```python
from build123d import *

# Parameters (mm, degrees)
IZIM1_W                     = 72
IZIM1_H                     = 72
Y_KSEKLIK_EKSTR_ZYON1_DEPTH = 340


with BuildPart() as part:
    # Çizim1 → Yükseklik-Ekstrüzyon1 (new body)
    with BuildSketch(Plane.XY):
        with BuildLine():
            Line((-36, 40), (36, 40))
            ThreePointArc((36, 40), (38.828427125, 38.828427125), (40, 36))
            Line((40, 36), (40, -36))
            ThreePointArc((40, -36), (38.828427125, -38.828427125), (36, -40))
            Line((36, -40), (-36, -40))
            ThreePointArc((-36, -40), (-38.828427125, -38.828427125), (-40, -36))
            Line((-40, -36), (-40, 36))
            ThreePointArc((-40, 36), (-38.828427125, 38.828427125), (-36, 40))
        make_face()
        Rectangle(IZIM1_W, IZIM1_H, mode=Mode.SUBTRACT)
    extrude(amount=Y_KSEKLIK_EKSTR_ZYON1_DEPTH)


solid = part.part
```
Geometry: final body of the model. Coordinates: model frame, mm. A direction names the side the tool comes from. Round coordinates to 2 decimals unless told otherwise and drop trailing zeros. Order: outer loops, then holes, each group sorted by start corner. A loop starts at its lowest first (then second) coordinate and runs counter-clockwise, first axis right, second up. Notation, with made-up numbers: (-7.75, 2) - (29.25, 2) arc R23 ccw to (29.25, 21) - close; hole circle Ø5 at (34.25, 77). An arc over 180 degrees is marked (long way). Write item = value, one per line. Start each with the question number.
Q1. Access query for faces 4 (the flat face through (40, 1, 168)), 5 (the flat face through (-1, 36, 168)). Directions: +Z, -Z, +X, -X, +Y, -Y. A direction counts if a zero-diameter tool reaches every point of the face in a straight line with its end or side. Return the directions, or none.
Q2. Ray query, line 1 (X direction, y = -7, z = 54); line 2 (Y direction, x = -37, z = 54). Return the intervals inside material, ascending. Write a range as from..to.
Q3. Cut plane A-A on x = 6.5. Return the cut outline in (y, z).
Q4. Pull-direction query (Y, two-part tool) for faces 1 (the flat face through (-1, -36, 168)), 2 (the flat face through (3, -38, 340)), 3 (the flat face through (-1, 40, 168)); classes: +Y half, -Y half, draft (parallel to the pull), parting line (faces both ways), or undercut.
Q5. Cut plane C-C on z = 216.5. Return the cut outline in (x, y), and give its area (3 significant figures).
Outcome:
q1.face_4 = +Z, -Z, +X, +Y, -Y
q1.face_5 = +Z, -Z
q2.line_1 = -40..-36, 36..40
q2.line_2 = -39.87..39.87
q3.outline = (-40, 0) - (-36, 0) - (-36, 340) - (-40, 340) - close; (36, 0) - (40, 0) - (40, 340) - (36, 340) - close
q4.face_1 = undercut
q4.face_2 = draft
q4.face_3 = +Y half
q5.outline = (-40, -36) arc R4 ccw to (-36, -40) - (36, -40) arc R4 ccw to (40, -36) - (40, 36) arc R4 ccw to (36, 40) - (-36, 40) arc R4 ccw to (-40, 36) - close; hole (-36, -36) - (36, -36) - (36, 36) - (-36, 36) - close
q5.area = 1,200 mm^2
